Input: part model. Units: mm. Frame: model coordinates. Coordinates: 2 decimals unless noted, no trailing zeros. Order: outer loops, then holes, each group sorted by start corner. A loop starts at its lowest first (then second) coordinate and runs counter-clockwise, first axis right, second up. Notation, with made-up numbers: (71.25, 28.5) - (89.25, 28.5) arc R26 cw to (89.25, 56.5) - close; hole circle Ø2 at (26.5, 69). An arc over 180 degrees is marked (long way). One line per question, with ' | ' between items.
from build123d import *

# Parameters (mm, degrees)
SKETCH1_W             = 76.2
SKETCH1_H             = 9.525
BOSS_EXTRUDE1_DEPTH   = 146.524999939
F_3_0MM_DOWEL_HOLE2_D = 3
FILLET1_R             = 1.27
F_6_0MM_DOWEL_HOLE2_D = 6


with BuildPart() as part:
    # Sketch1 → Boss-Extrude1 (new body, symmetric)
    with BuildSketch(Plane(origin=(0, 0, 0), x_dir=(0, 0, -1), z_dir=(1, 0, 0))):
        with Locations((0, 4.7625)):
            Rectangle(SKETCH1_W, SKETCH1_H)
    extrude(amount=BOSS_EXTRUDE1_DEPTH, both=True)

    # Ø3.0mm Dowel Hole2 (through all)
    with Locations(Plane(origin=(0, 9.525, 0), x_dir=(1, 0, 0), z_dir=(0, 1, 0))):
        with Locations((-137, 17.000000036), (-137, -17.000000036), (-68.5, 17.000000036), (-68.5, -17.000000036), (0, 17.000000036), (0, -17.000000036), (68.5, 17.000000036), (68.5, -17.000000036), (137, 17.000000036), (137, -17.000000036)):
            Hole(F_3_0MM_DOWEL_HOLE2_D / 2)

    # Fillet1
    fillet1_edges = [part.edges().sort_by_distance(p)[0] for p in [
        (0, 9.525, 38.1),
        (0, 9.525, -38.1),
        (0, 0, -38.1),
        (0, 0, 38.1),
    ]]
    fillet(fillet1_edges, radius=FILLET1_R)

    # Ø6.0mm Dowel Hole2 (through all)
    with Locations(Plane(origin=(0, 9.525, 0), x_dir=(1, 0, 0), z_dir=(0, 1, 0))):
        with Locations((-115.25, 12.5), (-115.25, -12.5), (-90.25, 12.5), (-90.25, -12.5), (90.25, 12.5), (90.25, -12.5), (115.25, 12.5), (115.25, -12.5)):
            Hole(F_6_0MM_DOWEL_HOLE2_D / 2)


solid = part.part
Item 1: Contact query for flat-ended pins moving along their axis: P1, Ø5.5, axis at x = -115.25, z = -12.5, coming from the -Y side; P2, Ø4, axis at x = 68.5, z = 17, coming from the -Y side. Output: stop coordinate, or through.
Data:
P1: through | P2: y = 0
Item 2: Ray query, line 1 (X direction, y = 4.5, z = -17) (3 decimals); line 2 (X direction, y = 4.5, z = -12) (3 decimals); line 3 (Z direction, x = -68.5, y = 2.75). Return the intervals inside material, ascending.
Data:
line 1: -146.525 to -138.5, -135.5 to -70, -67 to -1.5, 1.5 to 67, 70 to 135.5, 138.5 to 146.525 | line 2: -146.525 to -118.208, -112.292 to -93.208, -87.292 to 87.292, 93.208 to 112.292, 118.208 to 146.525 | line 3: -38.1 to -18.5, -15.5 to 15.5, 18.5 to 38.1
Item 3: Section B-B on x = 115.25. Return the cut outline in (y, z) (3 decimals).
Data:
outline: (0, -36.83) arc R1.27 ccw to (1.27, -38.1) - (8.255, -38.1) arc R1.27 ccw to (9.525, -36.83) - (9.525, -15.5) - (0, -15.5) - close; (0, -9.5) - (9.525, -9.5) - (9.525, 9.5) - (0, 9.5) - close; (0, 15.5) - (9.525, 15.5) - (9.525, 36.83) arc R1.27 ccw to (8.255, 38.1) - (1.27, 38.1) arc R1.27 ccw to (0, 36.83) - close
Item 4: Section A-A on z = 12.5. Return the cut outline in (x, y) (3 decimals), and give its area (3 significant figures).
Data:
outline: (-146.525, 0) - (-118.25, 0) - (-118.25, 9.525) - (-146.525, 9.525) - close; (-112.25, 0) - (-93.25, 0) - (-93.25, 9.525) - (-112.25, 9.525) - close; (-87.25, 0) - (87.25, 0) - (87.25, 9.525) - (-87.25, 9.525) - close; (93.25, 0) - (112.25, 0) - (112.25, 9.525) - (93.25, 9.525) - close; (118.25, 0) - (146.525, 0) - (146.525, 9.525) - (118.25, 9.525) - close | area: 2,560 mm^2
Item 5: Draft query along Z for faces 1 (the face through (146.525, 5, 1)), 2 (the face through (2, 5, -38.1)), 3 (the face through (112.39, 4.7, -13.4)). Return one class per face: released by +Z, released by -Z, zero draft, split by the parting line, or undercut.
Data:
face 1: zero draft | face 2: released by -Z | face 3: undercut
